Design review of the part built by this model. Coordinates are the model's own, in mm. A direction names the side the tool comes from. Give positions to 0.01 mm unless a question says otherwise; leave off trailing zeros. Loops run counter-clockwise (first coordinate to the right, second up) from the corner with the lowest first, then second, coordinate; pieces in that order, holes last. Notation, with made-up numbers: (50.5, -29.5) - (105.5, -29.5) arc R27 cw to (105.5, -5.5) - close; hole circle Ø11 at (52, 84.25). An arc over 180 degrees is marked (long way). Write each question's results on one line, items separated by ' | '.
from build123d import *

# Parameters (mm, degrees)
SKETCH_1_W             = 165
SKETCH_1_H             = 9
EXTRUDE_1_DEPTH        = 3
SKETCH_2_W             = 20
SKETCH_2_H             = 6
SKETCH_2_W_2           = 57
EXTRUDE_2_DEPTH        = 3
FILLET_1_R             = 2
SKETCH_3_W             = 12
SKETCH_3_H             = 3
CUT_EXTRUDE_1_DEPTH    = 87.113297463
SKETCH_5_R             = 1
CUT_EXTRUDE_3_DEPTH    = 87.113297463
EXTRUDE_4_DEPTH        = 3
SKETCH_10_R            = 1
CUT_EXTRUDE_5_DEPTH    = 93.841262378
CUT_EXTRUDE_6415_DEPTH = 93.841262378
FILLET_2_R             = 2
FILLET_3_R             = 10
CUT_EXTRUDE_6_DEPTH    = 93.841262378
FILLET_4_R             = 2
SKETCH_12_R            = 1.1
SKETCH_12_R_2          = 1.5
CUT_EXTRUDE_7_DEPTH    = 93.841262378


with BuildPart() as part:
    # 草图1 → 凸台-拉伸1 (new body)
    with BuildSketch(Plane(origin=(0, 0, 0), x_dir=(1, 0, 0), z_dir=(0, 1, 0))):
        Rectangle(SKETCH_1_W, SKETCH_1_H)
    extrude(amount=EXTRUDE_1_DEPTH)

    # 草图2 → 凸台-拉伸2 (add)
    with BuildSketch(Plane(origin=(0, 3, 0), x_dir=(1, 0, 0), z_dir=(0, 1, 0))):
        with Locations((-72.5, 7.5)):
            Rectangle(SKETCH_2_W, SKETCH_2_H)
        Polygon((82.5, -24.5), (82.5, -4.5), (25.5, -4.5), (76.5, -24.5), align=None)
        with Locations((54, 7.5)):
            Rectangle(SKETCH_2_W_2, SKETCH_2_H)
    extrude(amount=-EXTRUDE_2_DEPTH)

    # 圆角1
    fillet_1_edges = [part.edges().sort_by_distance(p)[0] for p in [
        (-82.5, 1.5, -10.5),
        (-62.5, 1.5, -10.5),
        (-62.5, 1.5, -4.5),
        (82.5, 1.5, -10.5),
        (25.5, 1.5, -4.5),
        (25.5, 1.5, -10.5),
        (-82.5, 1.5, 4.5),
    ]]
    fillet(fillet_1_edges, radius=FILLET_1_R)

    # 草图3 → 切除-拉伸1 (cut, through all)
    with BuildSketch(Plane(origin=(0, 3, 0), x_dir=(1, 0, 0), z_dir=(0, 1, 0))):
        with Locations((-72.5, 3)):
            Rectangle(SKETCH_3_W, SKETCH_3_H)
        with Locations((-34.5, 3)):
            Rectangle(SKETCH_3_W, SKETCH_3_H)
        with Locations((-2.5, 3)):
            Rectangle(SKETCH_3_W, SKETCH_3_H)
        with Locations((38, 3)):
            Rectangle(SKETCH_3_W, SKETCH_3_H)
        with Locations((70, 3)):
            Rectangle(SKETCH_3_W, SKETCH_3_H)
    extrude(amount=-CUT_EXTRUDE_1_DEPTH, mode=Mode.SUBTRACT)

    # 草图5 → 切除-拉伸3 (cut, through all)
    with BuildSketch(Plane(origin=(0, 3, 0), x_dir=(1, 0, 0), z_dir=(0, 1, 0))):
        with Locations((-67.5, 4.5)):
            Circle(SKETCH_5_R)
        with Locations((-67.5, 1.5)):
            Circle(SKETCH_5_R)
        with Locations((-77.5, 1.5)):
            Circle(SKETCH_5_R)
        with Locations((-77.5, 4.5)):
            Circle(SKETCH_5_R)
        with Locations((-29.5, 1.5)):
            Circle(SKETCH_5_R)
        with Locations((-39.5, 1.5)):
            Circle(SKETCH_5_R)
        with Locations((2.5, 1.5)):
            Circle(SKETCH_5_R)
        with Locations((-7.5, 1.5)):
            Circle(SKETCH_5_R)
        with Locations((33, 1.5)):
            Circle(SKETCH_5_R)
        with Locations((43, 1.5)):
            Circle(SKETCH_5_R)
        with Locations((43, 4.5)):
            Circle(SKETCH_5_R)
        with Locations((33, 4.5)):
            Circle(SKETCH_5_R)
        with Locations((75, 4.5)):
            Circle(SKETCH_5_R)
        with Locations((65, 4.5)):
            Circle(SKETCH_5_R)
        with Locations((65, 1.5)):
            Circle(SKETCH_5_R)
        with Locations((75, 1.5)):
            Circle(SKETCH_5_R)
    extrude(amount=-CUT_EXTRUDE_3_DEPTH, mode=Mode.SUBTRACT)

    # 草图9 → 凸台-拉伸4 (add)
    with BuildSketch(Plane(origin=(0, 3, 0), x_dir=(1, 0, 0), z_dir=(0, 1, 0))):
        Polygon((82.5, -15.5), (82.5, -24.5), (89.5, -24.5), (89.5, 4.5), (82.5, 4.5), (82.5, -3.5), (85.5, -3.5), (85.5, -15.5), align=None)
    extrude(amount=-EXTRUDE_4_DEPTH)

    # 草图10 → 切除-拉伸5 (cut, through all)
    with BuildSketch(Plane(origin=(0, 3, 0), x_dir=(1, 0, 0), z_dir=(0, 1, 0))):
        with Locations((85.5, -4.5)):
            Circle(SKETCH_10_R)
        with Locations((85.5, -14.5)):
            Circle(SKETCH_10_R)
        with Locations((82.5, -14.5)):
            Circle(SKETCH_10_R)
        with Locations((82.5, -4.5)):
            Circle(SKETCH_10_R)
    extrude(amount=-CUT_EXTRUDE_5_DEPTH, mode=Mode.SUBTRACT)

    # 草图6 → Cut-Extrude 6415 (cut, through all)
    with BuildSketch(Plane(origin=(0, 3, 0), x_dir=(1, 0, 0), z_dir=(0, 1, 0))):
        with BuildLine():
            Line((-78.6, 4.5), (-78.6, 1.5))
            ThreePointArc((-78.6, 1.5), (-77.550051841, 0.401139311), (-76.404554885, 1.4))
            Line((-76.404554885, 1.4), (-68.595445115, 1.4))
            ThreePointArc((-68.595445115, 1.4), (-67.449948159, 0.401139311), (-66.4, 1.5))
            Line((-66.4, 1.5), (-66.4, 4.5))
            ThreePointArc((-66.4, 4.5), (-67.449948159, 5.598860689), (-68.595445115, 4.6))
            Line((-68.595445115, 4.6), (-76.404554885, 4.6))
            ThreePointArc((-76.404554885, 4.6), (-77.550051841, 5.598860689), (-78.6, 4.5))
        make_face()
        with BuildLine():
            Line((34.095445115, 4.6), (41.904554885, 4.6))
            ThreePointArc((41.904554885, 4.6), (43.050051841, 5.598860689), (44.1, 4.5))
            Line((44.1, 4.5), (44.1, 1.5))
            ThreePointArc((44.1, 1.5), (43.050051841, 0.401139311), (41.904554885, 1.4))
            Line((41.904554885, 1.4), (34.095445115, 1.4))
            ThreePointArc((34.095445115, 1.4), (32.949948159, 0.401139311), (31.9, 1.5))
            Line((31.9, 1.5), (31.9, 4.5))
            ThreePointArc((31.9, 4.5), (32.949948159, 5.598860689), (34.095445115, 4.6))
        make_face()
        with BuildLine():
            Line((63.9, 4.5), (63.9, 1.5))
            ThreePointArc((63.9, 1.5), (64.949948159, 0.401139311), (66.095445115, 1.4))
            Line((66.095445115, 1.4), (73.904554885, 1.4))
            ThreePointArc((73.904554885, 1.4), (75.050051841, 0.401139311), (76.1, 1.5))
            Line((76.1, 1.5), (76.1, 4.5))
            ThreePointArc((76.1, 4.5), (75.050051841, 5.598860689), (73.904554885, 4.6))
            Line((73.904554885, 4.6), (66.095445115, 4.6))
            ThreePointArc((66.095445115, 4.6), (64.949948159, 5.598860689), (63.9, 4.5))
        make_face()
        with BuildLine():
            Line((-38.404554885, 4.6), (-30.595445115, 4.6))
            ThreePointArc((-30.595445115, 4.6), (-29.449948159, 5.598860689), (-28.4, 4.5))
            Line((-28.4, 4.5), (-28.4, 1.5))
            ThreePointArc((-28.4, 1.5), (-29.449948159, 0.401139311), (-30.595445115, 1.4))
            Line((-30.595445115, 1.4), (-38.404554885, 1.4))
            ThreePointArc((-38.404554885, 1.4), (-39.550051841, 0.401139311), (-40.6, 1.5))
            Line((-40.6, 1.5), (-40.6, 4.5))
            ThreePointArc((-40.6, 4.5), (-39.550051841, 5.598860689), (-38.404554885, 4.6))
        make_face()
        with BuildLine():
            Line((-8.6, 4.5), (-8.6, 1.5))
            ThreePointArc((-8.6, 1.5), (-7.550051841, 0.401139311), (-6.404554885, 1.4))
            Line((-6.404554885, 1.4), (1.404554885, 1.4))
            ThreePointArc((1.404554885, 1.4), (2.550051841, 0.401139311), (3.6, 1.5))
            Line((3.6, 1.5), (3.6, 4.5))
            ThreePointArc((3.6, 4.5), (2.550051841, 5.598860689), (1.404554885, 4.6))
            Line((1.404554885, 4.6), (-6.404554885, 4.6))
            ThreePointArc((-6.404554885, 4.6), (-7.550051841, 5.598860689), (-8.6, 4.5))
        make_face()
        with BuildLine():
            Line((82.48, -5.519803903), (82.48, -13.480196097))
            ThreePointArc((82.48, -13.480196097), (81.480049025, -14.510000481), (82.5, -15.52))
            Line((82.5, -15.52), (85.5, -15.52))
            ThreePointArc((85.5, -15.52), (86.519950975, -14.510000481), (85.52, -13.480196097))
            Line((85.52, -13.480196097), (85.52, -5.519803903))
            ThreePointArc((85.52, -5.519803903), (86.519950975, -4.489999519), (85.5, -3.48))
            Line((85.5, -3.48), (82.5, -3.48))
            ThreePointArc((82.5, -3.48), (81.480049025, -4.489999519), (82.48, -5.519803903))
        make_face()
    extrude(amount=-CUT_EXTRUDE_6415_DEPTH, mode=Mode.SUBTRACT)

    # 圆角2
    fillet_2_edges = [part.edges().sort_by_distance(p)[0] for p in [
        (89.5, 1.5, 24.5),
        (89.5, 1.5, -4.5),
        (82.5, 1.5, -4.5),
    ]]
    fillet(fillet_2_edges, radius=FILLET_2_R)

    # 圆角3
    fillet_3_edges = [part.edges().sort_by_distance(p)[0] for p in [
        (76.5, 1.5, 24.5),
        (25.5, 1.5, 4.5),
    ]]
    fillet(fillet_3_edges, radius=FILLET_3_R)

    # 草图11 → 切除-拉伸6 (cut, through all)
    with BuildSketch(Plane(origin=(0, 3, 0), x_dir=(1, 0, 0), z_dir=(0, 1, 0))):
        Polygon((34.16127674, -3.6), (77.5, -3.6), (77.5, -20.595577749), align=None)
    extrude(amount=-CUT_EXTRUDE_6_DEPTH, mode=Mode.SUBTRACT)

    # 圆角4
    fillet_4_edges = [part.edges().sort_by_distance(p)[0] for p in [
        (77.5, 1.5, 20.595577749),
        (34.16127674, 1.5, 3.6),
        (77.5, 1.5, 3.6),
    ]]
    fillet(fillet_4_edges, radius=FILLET_4_R)

    # 草图12 → 切除-拉伸7 (cut, through all)
    with BuildSketch(Plane(origin=(0, 3, 0), x_dir=(1, 0, 0), z_dir=(0, 1, 0))):
        with Locations(Location((-68.5, 7.5, 0), (0, 0, 270))):
            Circle(SKETCH_12_R)
        with Locations(Location((31.5, 7.5, 0), (0, 0, 270))):
            Circle(SKETCH_12_R)
        with Locations(Location((35, -5.5, 0), (0, 0, 270))):
            Circle(SKETCH_12_R_2)
        with Locations((-72, -5.5)):
            Circle(SKETCH_12_R_2)
    extrude(amount=-CUT_EXTRUDE_7_DEPTH, mode=Mode.SUBTRACT)


solid = part.part
(1) Wall thickness on line 1 along X through (y, z) = (2, -7.5); line 2 along Z through (x, y) = (-68.5, 0.95); line 3 along Z through (x, y) = (43, 0.7): over which ranges is each line inside the solid? List them lowest first. Write a range as from..to.
Answers below:
line 1: -82.5..-69.6, -67.4..-62.5, 25.5..30.4, 32.6..82.5 | line 2: -10.5..-8.6, -6.4..-4.96, -1.04..4.5 | line 3: -10.5..-5.6, -0.4..4.61, 6.59..11.36
(2) Take a section at B-B on y = 2. Count the separate pieces of the cut face and the enclosed holes in it, plus the area to 3 significant figures.
Answers below:
separate pieces: 1 | enclosed holes: 8 | area: 2,150 mm2
(3) Draft analysis for pull direction X (two halves, no side actions). For faces 4 (the flat face through (-51, 1, -4.5)), 5 (the flat face through (-73, 2, -10.5)), 6 (the cylindrical face through (76.604, 1.479, 19.33)), 7 (the cylindrical face through (25.49, 1.48, 4.68)), state which applies: pulls with the +X half, pulls with the -X half, needs draft (parallel to the pull), parting line crosses it, or undercut.
Answers below:
face 4: undercut | face 5: needs draft | face 6: undercut | face 7: pulls with the -X half
(4) Take a section at A-A on z = 10.5. Give the boundary of the cut face in (x, y).
Answers below:
outline: (40.8, 0) - (51.76, 0) - (51.76, 3) - (40.8, 3) - close; (77.5, 0) - (82.48, 0) - (82.48, 3) - (77.5, 3) - close; (85.52, 0) - (89.5, 0) - (89.5, 3) - (85.52, 3) - close
(5) Take a section at C-C on x = -17. Give the boundary of the cut face in (y, z).
Answers below:
outline: (0, -4.5) - (3, -4.5) - (3, 4.5) - (0, 4.5) - close
(6) Insertion check: P1, Ø1.5, axis at x = 60.5, y = 2, coming from the +Z side; P2, Ø1, axis at x = 39, y = 0.5, coming from the +Z side; P3, Ø1, axis at y = 1, z = -8, coming from the +X side; P4, Ø2, axis at x = 12.5, z = 3.5, coming from the -Y side. Each pin has a flat end and moves straight along its axis. Give the tip position at first contact, or say it passes through.
Answers below:
P1: z = 18.52 | P2: z = 9.99 | P3: x = 82.5 | P4: y = 0
(7) Tool access review of faces 1 (the flat face through (85.52, 2, 10)), 2 (the flat face through (83, 2, 24.5)), 3 (the flat face through (-40.6, 2, -3)): name each direction out of +Z, -Z, +X, -X, +Y, -Y from which nothing blocks a thin tool from reaching the whole face with its end or side.
Answers below:
face 1: +Y, -Y | face 2: +Z, +X, -X, +Y, -Y | face 3: -Z, +Y, -Y
